Input: dimensioned drawing with shaded views. Units: mm. Origin: part minimum x, y, z. A direction names the side the tool comes from. Round coordinates to 2 decimals unless told otherwise and drop trailing zeros. Write each loop counter-clockwise with the first axis right and the second up, starting at its lowest first coordinate (ties: lowest second). Pieces come first, ordered by that corner, then holes. Notation, with made-up numbers: M -18.5,80.25 L 12.5,80.25 A10 cw 12.5,97.25 Z; hole C -31.75,-33 d1. An arc over 180 degrees is marked long. Answer in a Markdown table with one row per item. Add a question column.
Item 1: Contact query for flat-ended pins moving along their axis: pin 1 (2 mm diameter, centred on x = 18, y = 0.5, fed in from -Z); pin 2 (0.8 mm diameter, centred on y = 4, z = 4.5, fed in from +X); pin 3 (0.8 mm diameter, centred on x = 16, y = 1, fed in from +Z). Output: stop coordinate, or through.
Item 2: Cut plane B-B on x = 2. Return loops of the section in (y, z).
Item 3: Set-up query: the marked faces 1, 2, 3, 4 and 5. Return all of +Z, -Z, +X, -X, +Y, -Y with unobstructed straight access to the full face (end or side cutting, diameter ignored); none if empty.
Item 4: Material intervals for probe 1 along Y at (x, z) = (12.75, 6.25); probe 2 along Z at (x, y) = (1.25, 2.6); probe 3 along Z at (x, y) = (1, 1.2), sorted ascending.
Item 5: Mould query, pull axis Z, two halves, no side actions, for the marked faces 6, 7 and 8. Classes: released by +Z, released by -Z, zero draft, split by the parting line, or undercut.
Item 6: Cut plane C-C on y = 1.95. Return loops of the section in (x, z) (1 decimal), and give its area (3 significant figures).
Item 7: Cut plane A-A on y = 3.55. Give the number of separate pieces and of enclosed holes in the cut face.
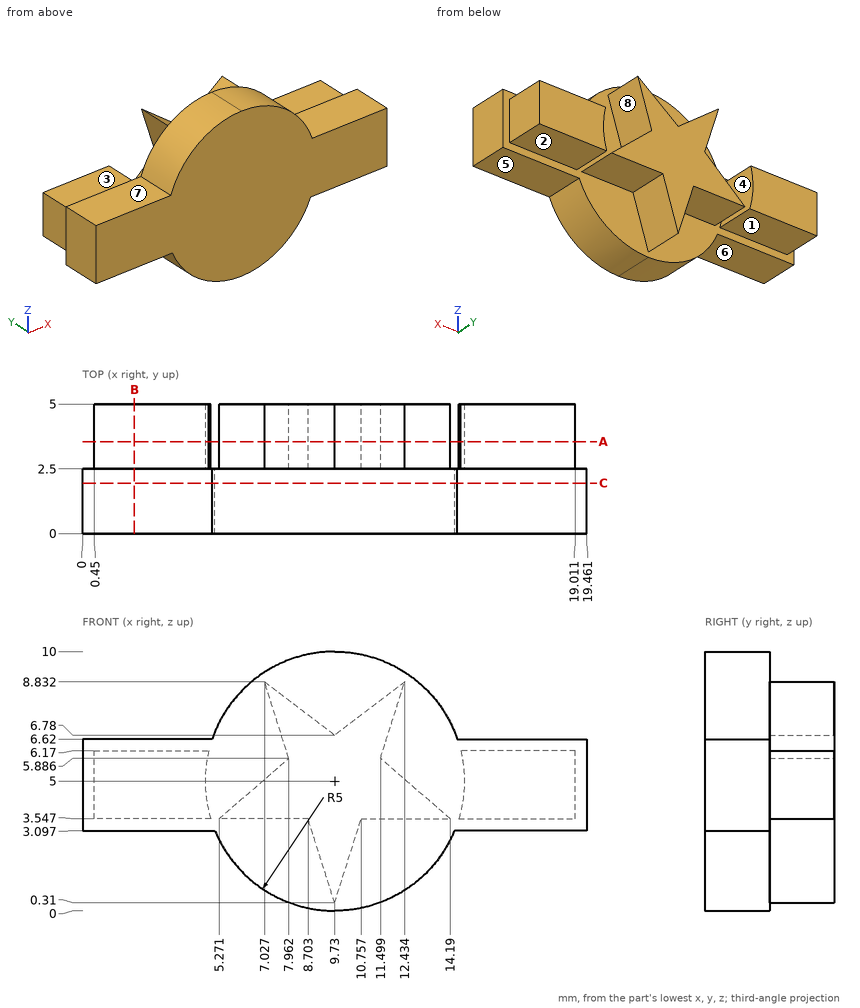
Results below:
| question | item | result |
|---|---|---|
| 1 | pin 1 | z = 3.1 |
| 1 | pin 2 | x = 19.01 |
| 1 | pin 3 | z = 6.62 |
| 2 | outline | M 0,3.1 L 2.5,3.1 L 2.5,3.55 L 5,3.55 L 5,6.17 L 2.5,6.17 L 2.5,6.62 L 0,6.62 Z |
| 3 | face 1 | -Z, -X, +Y |
| 3 | face 2 | -Z, +X, +Y |
| 3 | face 3 | +Z, -X, +Y |
| 3 | face 4 | +Y |
| 3 | face 5 | -Z, +X, +Y, -Y |
| 4 | probe 1 | 0 to 2.5 |
| 4 | probe 2 | 3.55 to 6.17 |
| 4 | probe 3 | 3.1 to 6.62 |
| 5 | face 6 | released by -Z |
| 5 | face 7 | released by +Z |
| 5 | face 8 | undercut |
| 6 | outline | M 0,3.1 L 5.1,3.1 A5 ccw 14.4,3.1 L 19.5,3.1 L 19.5,6.6 L 14.5,6.6 A5 ccw 5,6.6 L 0,6.6 Z |
| 6 | area | 113 mm2 |
| 7 | separate pieces | 3 |
| 7 | enclosed holes | 0 |
